```python
from build123d import *

# Parameters (mm, degrees)
CROQUIS1_R              = 5.275
SALIENTE_EXTRUIR1_DEPTH = 2
CROQUIS2_R              = 11.125
SALIENTE_EXTRUIR2_DEPTH = 6.05


with BuildPart() as part:
    # Croquis1 → Saliente-Extruir1 (new body)
    with BuildSketch(Plane(origin=(0, 0, 0), x_dir=(0, 0, -1), z_dir=(1, 0, 0))):
        with BuildLine():
            Line((60.7, 3.36816026), (60.7, 0))
            Line((60.7, 0), (60.7, -15))
            ThreePointArc((60.7, -15), (77.15, -31.45), (93.6, -15))
            Line((93.6, -15), (93.6, 0))
            Line((93.6, 0), (93.6, 3.36816026))
            Line((93.6, 3.36816026), (60.7, 3.36816026))
        make_face()
        with Locations((76.9, -15)):
            Circle(CROQUIS1_R, mode=Mode.SUBTRACT)
    extrude(amount=SALIENTE_EXTRUIR1_DEPTH)

    # Croquis2 → Saliente-Extruir2 (add)
    with BuildSketch(Plane(origin=(2, 0, 0), x_dir=(0, 0, -1), z_dir=(1, 0, 0))):
        with BuildLine():
            Line((93.6, -15), (93.6, 3.36816026))
            Line((93.6, 3.36816026), (60.7, 3.36816026))
            Line((60.7, 3.36816026), (60.7, -15))
            ThreePointArc((60.7, -15), (77.15, -31.45), (93.6, -15))
        make_face()
        with Locations((76.9, -15)):
            Circle(CROQUIS2_R, mode=Mode.SUBTRACT)
    extrude(amount=SALIENTE_EXTRUIR2_DEPTH)


solid = part.part
```
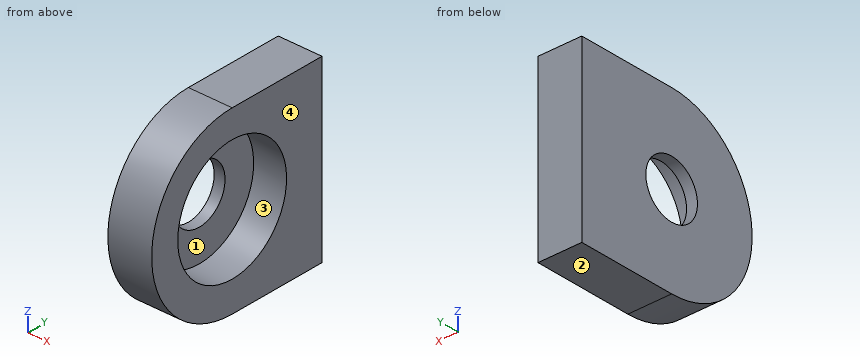
Source: CAD feature listing. Evaluate the final solid. Frame: model axes, mm. Face numbers are marked on the shaded views. Give positions to 0.01 mm unless a question says otherwise; leave off trailing zeros. Loops run counter-clockwise (first coordinate to the right, second up) from the corner with the lowest first, then second, coordinate; pieces in that order, holes last. Notation, with made-up numbers: (-18, 55.5) - (1, 55.5) arc R7 cw to (1, 66.5) - close; hole circle Ø4 at (-0.5, 70.25). An arc over 180 degrees is marked (long way). Use CSV: the item, a comma, the result in double quotes.
1) Line query: line 1 (Y direction, x = 0.65, z = -76.9) (3 decimals); line 2 (Y direction, x = 4.75, z = -76.9) (3 decimals); line 3 (X direction, y = -22, z = -80). Output: solid intervals per line, ascending.
Worked out:
line 1,"y = -31.448 to -20.275, -9.725 to 3.368"
line 2,"y = -31.448 to -26.125, -3.875 to 3.368"
line 3,"x = 0 to 2"
2) Mould query, pull axis Z, two halves, no side actions, for the marked faces 1, 2, 3 and 4. Classes: +Z half, -Z half, draft (parallel to the pull), parting line (faces both ways), or undercut.
Worked out:
face 1,"undercut"
face 2,"-Z half"
face 3,"undercut"
face 4,"draft"
3) Cut plane C-C (x = 2.75). Output: boundary loops of the cut face in (y, z) (3 decimals), and give its area (3 significant figures).
Worked out:
outline,"(-15, -93.6) - (3.368, -93.6) - (3.368, -60.7) - (-15, -60.7) arc R16.45 ccw to start; hole circle Ø22.25 at (-15, -76.9)"
area,"641 mm^2"
4) Cut plane A-A (z = -74). Output: boundary loops of the cut face in (x, y), and give its area (3 significant figures).
Worked out:
outline,"(0, -31.15) - (8.05, -31.15) - (8.05, -25.74) - (2, -25.74) - (2, -19.41) - (0, -19.41) - close; (0, -10.59) - (2, -10.59) - (2, -4.26) - (8.05, -4.26) - (8.05, 3.37) - (0, 3.37) - close"
area,"130 mm^2"
5) Cut plane D-D (z = -84). Output: boundary loops of the cut face in (x, y).
Worked out:
outline,"(0, -29.96) - (8.05, -29.96) - (8.05, -23.56) - (2, -23.56) - (2, -6.44) - (8.05, -6.44) - (8.05, 3.37) - (0, 3.37) - close"
6) Pin query (flat end, axial travel): P1, Ø3, axis at x = 4, z = -80, coming from the -Y side; P2, Ø2, axis at x = 5, y = -26.5, coming from the -Z side. Return the tip coordinate at first contact, or that it passes through.
Worked out:
P1,"stops at y = -31.39"
P2,"stops at z = -89.81"
7) Cut plane B-B (y = -18.5). Output: boundary loops of the cut face in (x, z).
Worked out:
outline,"(0, -93.22) - (8.05, -93.22) - (8.05, -87.46) - (2, -87.46) - (2, -80.85) - (0, -80.85) - close; (0, -72.95) - (2, -72.95) - (2, -66.34) - (8.05, -66.34) - (8.05, -61.08) - (0, -61.08) - close"
